Geometry: final body of the model. Coordinates: model frame, mm. A direction names the side the tool comes from. Give positions to 0.01 mm unless a question says otherwise; leave off trailing zeros. Loops run counter-clockwise (first coordinate to the right, second up) from the corner with the lowest first, then second, coordinate; pieces in that order, holes last.
1. Section A-A, the plane x = 6.25. Output: boundary loops of the cut face in (y, z), then the cut area to 3 significant figures.
2. Material intervals for line 1 along X through (y, z) = (1.75, 2.25); line 2 along Y through (x, z) = (-1, -0.75); line 3 along Z through (x, y) = (5.5, 0.5), sorted ascending.
3. First-contact query: P1, Ø4, axis at y = 1.5, z = -2, coming from the +X side; P2, Ø4, axis at x = 7.5, y = 1, coming from the +Z side; P3, Ø1, axis at x = 2.5, y = -1.5, coming from the +Z side; P4, Ø2, axis at x = 8.5, y = -2.5, coming from the -Z side. Flat tips, straight axial feed; report the tip coordinate or a pass-through.
4. Draft query along Y for faces 4 (the face through (-2, -1.25, 0)), 5 (the face through (6, 0, 2)), 6 (the face through (-2, 1.25, 0)), 7 (the face through (-2.8, -0.6, 1.3)). Return one class per face: +Y half, -Y half, draft (parallel to the pull), parting line (faces both ways), or undercut.
5. Access query for faces 1 (the face through (-1.217, 3.233, 1.341)), 2 (the face through (0, 2, -2)), 3 (the face through (-1.611, -0.616, 1.088)). Directions: +Z, -Z, +X, -X, +Y, -Y. A direction counts if a zero-diameter tool reaches every point of the face in a straight line with its end or side. Return the directions, or none.
Autodesk Inventor part; units mm, degrees
ref_plane "Work Plane1" through (29, 0, 0) normal (0, -1, 0) x (1, 0, 0)
ref_plane "YZ Plane" through (0, 0, 0) normal (1, 0, 0) x (0, 1, 0)
ref_plane "XZ Plane" through (0, 0, 0) normal (0, 1, 0) x (-1, 0, 0)
sketch "Sketch1" plane through (0, 0, 0) normal (0, 0, 1) x (1, 0, 0)
  line L0 (0.3333, 0) -> (12, 0)
  line L1 (12, 0) -> (12, 2)
  line L2 (12, 2) -> (2.1, 2)
  line L3 (2.1, 2) -> (1.6705, 2)
  line L4 (1.6705, 2) -> (0, 2)
  line L5 (0, 2) -> (0, 3.5)
  line L6 (0, 3.5) -> (-2.8, 3.5)
  line L7 (-2.8, 3.5) -> (-2.8, 1.4434)
  line L8 (-2.8, 1.4434) -> (-0.5, 1.4434)
  line L9 (-0.5, 1.4434) -> (0.3333, 0)
  line L10 (-5.76, 0) -> (14.96, 0)
  line L11 (0, -0.7) -> (0, 4.2)
  line L12 (2.1, 2) -> (0, 2) construction
  dimension "d1" = 9.9
  dimension "d2" = 0.4295
  dimension "d3" = 2.8
  dimension "d4" = 2.3
  dimension "d5" = 60
  dimension "d6" = 4
  dimension "d7" = 4
  dimension "d8" = 2.8868
  dimension "d9" = 7
  dimension "d26" = 12
revolve "Body" add sketch "Sketch1" angle 360 about axis through (0.3333, 0, 0) along (1, 0, 0) contours L9 L11 L4 L3 L2 L1 L0 | L9 L8 L7 L6 L5 L11
sketch "Sketch2" plane through (-2.8, 0, 0) normal (-1, 0, 0) x (0, 0, 1)
  circle A0 centre (0, 0) radius 1.4434
  line L0 (0, -4.9) -> (0, 4.9)
  line L1 (-4.9, 0) -> (4.9, 0)
  line L2 (1.4434, 0) -> (0.7217, -1.25)
  line L3 (0.7217, -1.25) -> (-0.7217, -1.25)
  line L4 (-0.7217, -1.25) -> (-1.4434, 0)
  line L5 (-1.4434, 0) -> (-0.7217, 1.25)
  line L6 (-0.7217, 1.25) -> (0.7217, 1.25)
  line L7 (0.7217, 1.25) -> (1.4434, 0)
  point P0 (0, 0)
extrude "Slot" add sketch "Sketch2" against normal up to next contours L7 A0 | A0 L2 | L6 L0 A0 | A0 L0 L3 | L0 L6 A0 | A0 L3 L0 | L4 A0 | A0 L5
fillet "Fillet1" radius 0.4 1 edges at (-2.8, -3.5, 0)
thread "Thread"
chamfer "Chamfer1" distance 0.4294 distance2 0.4294 1 edges at (12, -2, 0) measured on face at (12, -1.1003, -0.6618)
ref_plane "Work Plane1" through (29, 0, 0) normal (0, -1, 0) x (1, 0, 0)
fillet "Fillet2" radius 0.1 1 edges at (0, -2, 0)
equation "\"d1\" = GEL"
equation "\"d3\" = KOH"
equation "\"d4\" = INTI"
equation "\"d6\" = GD"
equation "\"d7\" = BDM"
equation "\"d8\" = 1.1547 * SW"
equation "\"d9\" = KOD"
equation "\"d26\" = NLG"
equation "\"d30\" = R"
equation "\"d17\" = RR"
equation "\"d13\" = GEL"
equation "\"d15\" = -0.5 * SPD + 0.5 * GD"
equation "\"d16\" = GUL"
equation "\"GD\" = NND"
equation "\"NLG\" = 12"
equation "\"GEL\" = 9.9"
equation "\"KOD\" = 7"
equation "\"KOH\" = 2.8"
equation "\"INTI\" = 2.3"
equation "\"GAL\" = 0.61345 * PTC"
equation "\"GUL\" = 0.61345 * PTC"
equation "\"BDM\" = NND"
equation "\"SW\" = 2.5"
equation "\"RR\" = 0.4"
equation "\"SPD\" = NND - 1.2269 * PTC"
equation "\"R\" = 0.1"
equation "\"TOA\" = 30deg"
equation "\"GD1\" = THREADDIA - 1.2269 * PTC"
equation "\"THREADDIA\" = 4"
equation "\"FAWI\" = 45deg"
equation "\"ANG\" = 120deg"
equation "\"PTC\" = 0.7"
equation "\"NND\" = 4"
equation "\"E0\" = 1.155 * SW"
properties part number "DIN 7984 - M4 x 12" material "Steel, Mild"
Answers below:
1. outline: circle Ø4 at (0, 0)
1. area: 12.6 mm2
2. line 1: x = -2.8 to 0
2. line 2: y = -3.42 to -1.2, 1.2 to 3.42
2. line 3: z = -1.94 to 1.94
3. P1: stops at x = 12
3. P2: stops at z = 2
3. P3: stops at z = 1.73
3. P4: stops at z = -1.32
4. face 4: undercut
4. face 5: parting line
4. face 6: undercut
4. face 7: draft
5. face 1: +X, -X
5. face 2: +X
5. face 3: -X
